Drawing for the job (mm, zero at the part's lowest x, y, z). A direction names the side the tool comes from. Round coordinates to 2 decimals unless told otherwise and drop trailing zeros. Write each loop counter-clockwise with the first axis right and the second up, starting at its lowest first coordinate (ties: lowest second). Pieces come first, ordered by that corner, then holes.
Item 1: Mould opens along X. For the marked faces 1, 2, 3 and 4 say: +X half, -X half, draft (parallel to the pull), parting line (faces both ways), or undercut.
Item 2: Band-saw the part on C-C, the plane x = 45. Write the cut outline in (y, z).
Item 3: Band-saw the part on A-A, the plane y = 85. Write the cut outline in (x, z), then the cut area to 3 significant figures.
Item 4: Wall check: probe 1 along Y at (x, z) = (15, 93); probe 2 along Y at (x, z) = (23.5, 19.5); probe 3 along Z at (x, y) = (15, 6). Give the ranges that are in metal, low to high.
Item 5: Band-saw the part on D-D, the plane z = 66.5. Write the cut outline in (x, y).
Item 6: Drop flat-ended pins along their axis: pin 1 Ø12 at (x, y) = (14, 55.5) entering from +Z; pin 2 Ø10 at (x, y) = (16.5, 88.5) entering from +Z; pin 3 Ø4 at (x, z) = (87.5, 20.5) entering from +Y. Give the stop position or say it passes through.
Item 7: Band-saw the part on B-B, the plane x = 89.5. Write the cut outline in (y, z).
Item 8: 3-axis set-ups, long thin cutter, end or side, ignore diameter. For the marked faces 5 and 6: which of +Z, -Z, +X, -X, +Y, -Y reach the whole face in a straight line?
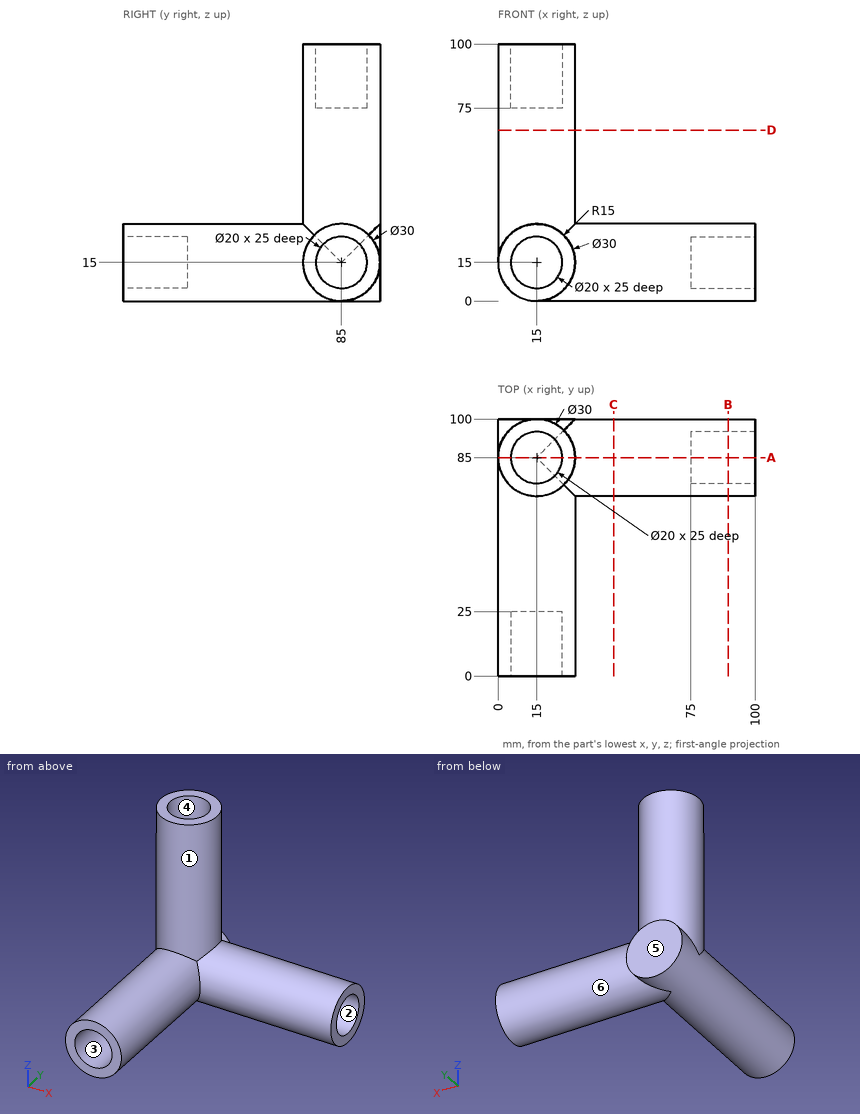
Results:
1. face 1: parting line
1. face 2: draft
1. face 3: undercut
1. face 4: undercut
2. outline: circle Ø30 at (85, 15)
3. outline: (0, 15) arc R15 ccw to (15, 0) - (100, 0) - (100, 5) - (75, 5) - (75, 25) - (100, 25) - (100, 30) - (30, 30) - (30, 100) - (25, 100) - (25, 75) - (5, 75) - (5, 100) - (0, 100) - close
3. area: 4,050 mm2
4. probe 1: y = 70 to 75, 95 to 100
4. probe 2: y = 25 to 100
4. probe 3: z = 0 to 5, 25 to 30
5. outline: circle Ø30 at (15, 85)
6. pin 1: stops at z = 30
6. pin 2: stops at z = 75
6. pin 3: stops at y = 99.59
7. outline: circle Ø30 at (85, 15); hole circle Ø20 at (85, 15)
8. face 5: +Z, -Z, +X, -X, +Y
8. face 6: +X
